Verification items for this drawing (mm, ordinates from the low corner). A direction names the side the tool comes from. Give positions to 0.01 mm unless a question says otherwise; leave off trailing zeros. Write each loop counter-clockwise with the first axis right and the second up, starting at its lowest first coordinate (ties: lowest second). Pieces come first, ordered by that corner, then holes. Notation, with made-up numbers: (88.5, 38.5) -> (129.5, 38.5) arc R36 cw to (129.5, 73.5) -> close; hole circle Ø9 at (82.5, -28). An arc over 180 degrees is marked (long way). One line per item, written item: value.
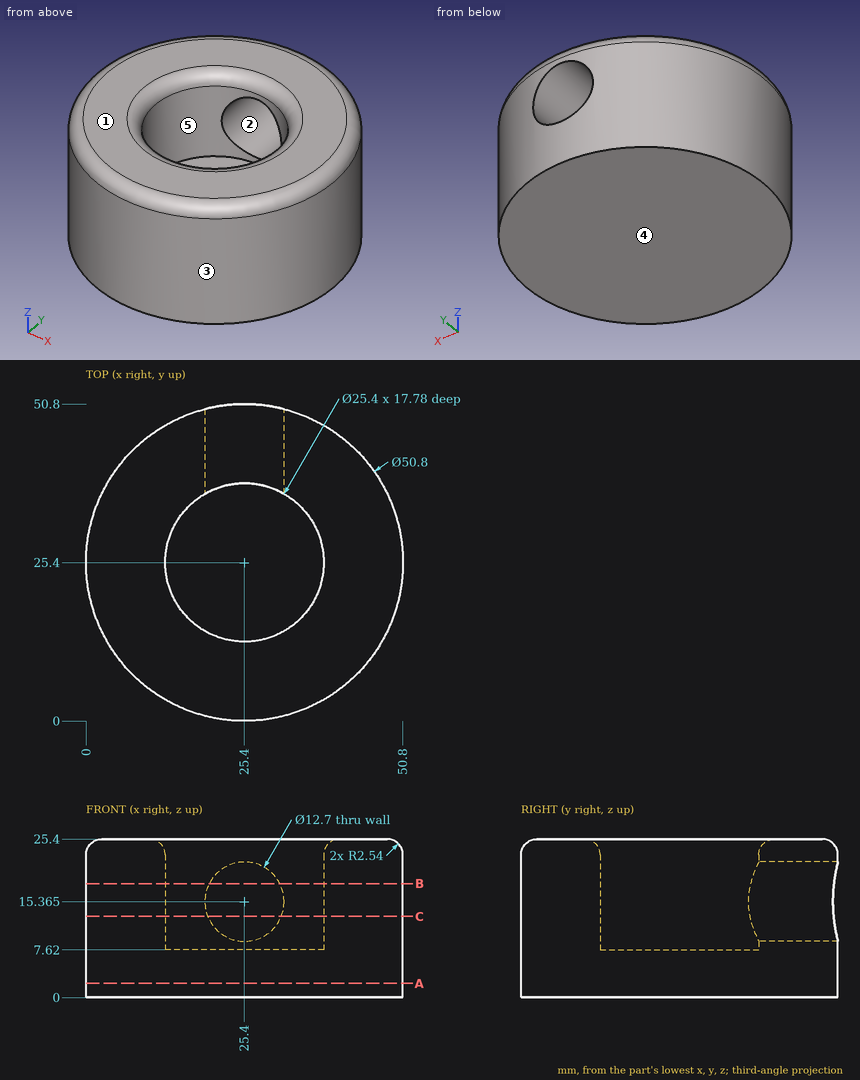
1) Sectioned sample at A-A on z = 2.25. Record the cut outline in (x, y), plus the area to 3 significant figures.
Verdict:
outline: circle Ø50.8 at (25.4, 25.4)
area: 2,030 mm^2
2) Mould release check, pull along X, two halves, no side actions. Record for the marked faces 3, 4 and 5: released by +X, released by -X, zero draft, split by the parting line, or undercut.
Verdict:
face 3: split by the parting line
face 4: zero draft
face 5: undercut
3) Depth check by flat-ended pin: pin 1 Ø10 at (y, z) = (38, 8) entering from +X; pin 2 Ø2 at (x, z) = (14, 9.5) entering from -Y; pin 3 Ø6 at (x, z) = (9.5, 7) entering from +Y; pin 4 Ø5 at (x, y) = (22, 38.5) entering from +Z. Enter the tip coordinate at first touch or a pass-through.
Verdict:
pin 1: x = 49.64
pin 2: y = 2.23
pin 3: y = 47.28
pin 4: z = 25.4
4) Scan lines: probe 1 along Y at (x, z) = (25.4, 18.75); probe 2 along X at (y, z) = (18, 12.75); probe 3 along X at (y, z) = (39.5, 11). Record each from-to range of solid material in increasing order.
Verdict:
probe 1: 0 to 12.7
probe 2: 1.1 to 15.08, 35.72 to 49.7
probe 3: 4.27 to 20.79, 30.01 to 46.53
5) Tool access check on the marked faces 1 and 2. Record the directions out of +Z, -Z, +X, -X, +Y, -Y that give a thin tool (end or side, any length) a straight path to the whole face; none if there is none.
Verdict:
face 1: +Z, +X, -X, +Y, -Y
face 2: +Y
6) Sectioned sample at C-C on z = 13. Record the cut outline in (x, y), plus the area to 3 significant figures.
Verdict:
outline: (19.51, 36.65) -> (19.51, 50.11) arc R25.4 ccw (long way) to (31.29, 50.11) -> (31.29, 36.65) arc R12.7 cw (long way) to start
area: 1,370 mm^2
7) Sectioned sample at B-B on z = 18.25. Record the cut outline in (x, y), plus the area to 3 significant figures.
Verdict:
outline: (19.74, 36.77) -> (19.74, 50.16) arc R25.4 ccw (long way) to (31.06, 50.16) -> (31.06, 36.77) arc R12.7 cw (long way) to start
area: 1,370 mm^2
